CAD build for the part. Positions are in the model's coordinates, mm. Face numbers are marked on the shaded views. A direction names the side the tool comes from. Round coordinates to 2 decimals unless told otherwise and drop trailing zeros. Loops run counter-clockwise (first coordinate to the right, second up) from the corner with the lowest first, then second, coordinate; pieces in that order, holes last. Notation, with made-up numbers: (77.25, 37.5) -> (85.25, 37.5) arc R12 cw to (85.25, 45.5) -> close; hole circle Ø7 at (61.5, 79.25). An arc over 180 degrees is marked (long way). Answer as CSV lines item,"result".
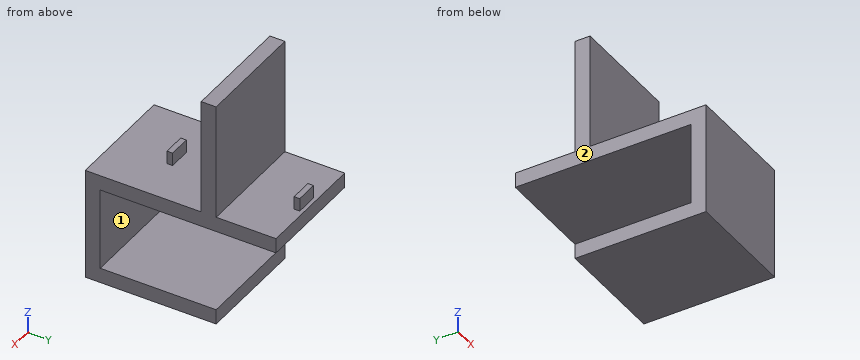
```python
from build123d import *

# Parameters (mm, degrees)
F0_W     = 62
F0_H     = 8
F1_DEPTH = 60
F2_W     = 12
F2_H     = 3
F3_DEPTH = 15
F4_W     = 8
F4_H     = 62
F4_W_2   = 32
F4_H_2   = 8
F5_DEPTH = 60
F6_W     = 12
F6_H     = 3
F7_DEPTH = 15


with BuildPart() as f1:
    # F0 (on Right) → F1 (new body)
    with BuildSketch(Plane.YZ):
        Polygon((129.916325, 0), (129.916325, 70), (121.916325, 70), (121.916325, 8), (121.916325, 0), align=None)
        Polygon((121.916325, 0), (121.916325, 8), (59.916325, 8), (59.916325, 0), (67.916325, 0), align=None)
        Polygon((67.916325, -44), (67.916325, 0), (59.916325, 0), (59.916325, -52), (67.916325, -52), align=None)
        with Locations((98.916325, -48)):
            Rectangle(F0_W, F0_H)
    extrude(amount=F1_DEPTH)

    # F2 (on Top) → F3 (join)
    with BuildSketch(Plane.XY):
        with Locations((30, 90.416325)):
            Rectangle(F2_W, F2_H)
    extrude(amount=F3_DEPTH)

    # F4 (on Right) → F5 (join)
    with BuildSketch(Plane.YZ):
        with Locations((125.916325, 39)):
            Rectangle(F4_W, F4_H)
        with Locations((145.916325, 4)):
            Rectangle(F4_W_2, F4_H_2)
        with Locations((125.916325, 4)):
            Rectangle(F4_W, F4_H_2)
        Polygon((121.916325, 0), (121.916325, 8), (59.916325, 8), (59.916325, -52), (129.916325, -52), (129.916325, -44), (67.916325, -44), (67.916325, 0), align=None)
    extrude(amount=F5_DEPTH)

    # F6 (on Top) → F7 (join)
    with BuildSketch(Plane.XY):
        with Locations((30, 158.416325)):
            Rectangle(F6_W, F6_H)
    extrude(amount=F7_DEPTH)


solid = f1.part
```
Q1. Drop flat-ended pins along their axis: pin 1 Ø3.5 at (x, y) = (27.5, 90.5) entering from +Z; pin 2 Ø0.9 at (y, z) = (158, 11) entering from -X; pin 3 Ø5 at (x, y) = (28.5, 149.5) entering from -Z. Give the stop position or say it passes through.
Results:
pin 1,"z = 15"
pin 2,"x = 24"
pin 3,"z = 0"
Q2. Tool access for the marked faces 1 and 2: list every direction of +Z, -Z, +X, -X, +Y, -Y with a clear straight run to the whole face (end or side of a thin tool).
Results:
face 1,"+X, -X, +Y"
face 2,"+Z, -Z, -X, +Y, -Y"
Q3. Slice it at D-D, the plane x = 8.5. Give the cut face in (y, z), and give its area (3 significant figures).
Results:
outline,"(59.92, -52) -> (129.92, -52) -> (129.92, -44) -> (67.92, -44) -> (67.92, 0) -> (161.92, 0) -> (161.92, 8) -> (129.92, 8) -> (129.92, 70) -> (121.92, 70) -> (121.92, 8) -> (59.92, 8) -> close"
area,"2,220 mm2"
Q4. Probe L1, parallel to Z at x = 55, y = 127.5; L2, parallel to Z at x = 29, y = 99; L3, parallel to Y at x = 32, z = 10. List the from-to ranges inside material, lowest first. Write a range as [from, to].
Results:
L1,"[-52, -44], [0, 70]"
L2,"[-52, -44], [0, 8]"
L3,"[88.92, 91.92], [121.92, 129.92], [156.92, 159.92]"
Q5. Slice it at A-A, the plane y = 73. Give the cut face in (x, z), and give its area (3 significant figures).
Results:
outline,"(0, -52) -> (60, -52) -> (60, -44) -> (0, -44) -> close; (0, 0) -> (60, 0) -> (60, 8) -> (0, 8) -> close"
area,"960 mm2"
Q6. Slice it at B-B, the plane x = 33. Give the cut face in (y, z), and give its area (3 significant figures).
Results:
outline,"(59.92, -52) -> (129.92, -52) -> (129.92, -44) -> (67.92, -44) -> (67.92, 0) -> (161.92, 0) -> (161.92, 8) -> (159.92, 8) -> (159.92, 15) -> (156.92, 15) -> (156.92, 8) -> (129.92, 8) -> (129.92, 70) -> (121.92, 70) -> (121.92, 8) -> (91.92, 8) -> (91.92, 15) -> (88.92, 15) -> (88.92, 8) -> (59.92, 8) -> close"
area,"2,270 mm2"
Q7. Slice it at C-C, the plane z = 45. Give the cut face in (x, y).
Results:
outline,"(0, 121.92) -> (60, 121.92) -> (60, 129.92) -> (0, 129.92) -> close"
